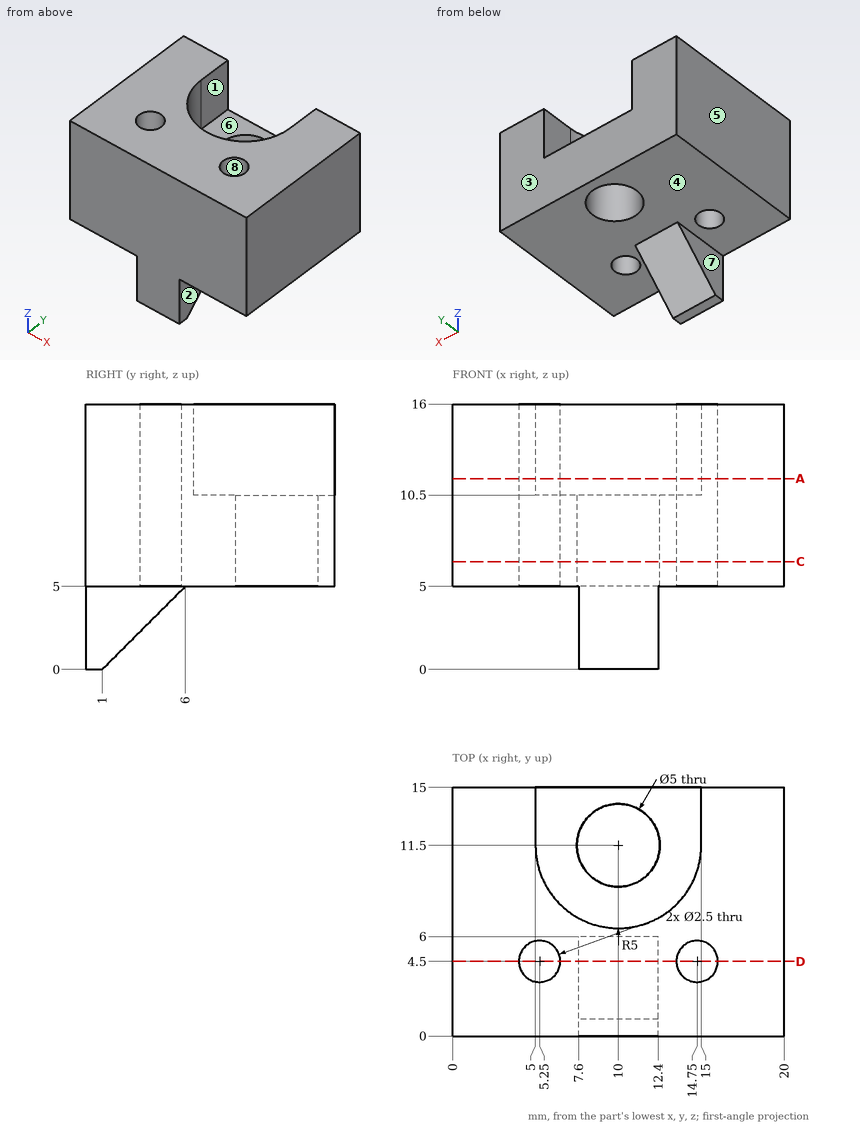
Can you work these out from the drawing? Everything is in mm from the part's minimum corner. A direction names the side the tool comes from. Round coordinates to 2 decimals unless told otherwise and drop trailing zeros. Loops run counter-clockwise (first coordinate to the right, second up) from the corner with the lowest first, then second, coordinate; pieces in that order, holes last. Notation, with made-up numbers: (42, -26) - (60, -26) arc R35 cw to (60, 11) - close; hole circle Ø7 at (-25, 8.25). An arc over 180 degrees is marked (long way). One line per question, with ' | ' between items. Start each with the question number.
Q1. I want a section at A-A (z = 11.5). Write out the boundary of the cut face in (x, y).
Q2. For the marked faces 4, 5, 6, 7 and 8, which set-ups out of +Z, -Z, +X, -X, +Y, -Y let a thin tool reach every point of the face, with its end or its side?
Q3. I want a section at D-D (y = 4.5). Write out the boundary of the cut face in (x, z), then the cut area to 3 significant figures.
Q4. Will these pins go through, and if not, where does the flat tip stop? pin 1 (1.5 mm diameter, centred on x = 5, y = 8, fed in from -Z); pin 2 (2.5 mm diameter, centred on y = 4, z = 2, fed in from +X); pin 3 (4 mm diameter, centred on x = 11.5, y = 9.5, fed in from +Z).
Q5. We'd pull the mould along X, two halves only. Please class the marked faces 1, 2 and 3: +X half, -X half, draft (parallel to the pull), parting line (faces both ways), or undercut.
Q6. I want a section at C-C (z = 6.5). Write out the boundary of the cut face in (x, y), then the cut area to 3 significant figures.
Q7. Please list where these lines run through material, in increasing order: line 1 (X direction, y = 11.5, z = 8.1); line 2 (Y direction, x = 10, z = 6.2); line 3 (Y direction, x = 5.25, z = 9). Write a range as [from, to].
Response values:
1) outline: (0, 0) - (20, 0) - (20, 15) - (15, 15) - (15, 11.5) arc R5 cw to (5, 11.5) - (5, 15) - (0, 15) - close; hole circle Ø2.5 at (5.25, 4.5); hole circle Ø2.5 at (14.75, 4.5)
2) face 4: -Z, +Y | face 5: +Z, -Z, -X, +Y, -Y | face 6: +Z, +Y | face 7: -Z, -X, +Y, -Y | face 8: +Z, -Z
3) outline: (0, 5) - (4, 5) - (4, 16) - (0, 16) - close; (6.5, 5) - (7.6, 5) - (7.6, 3.5) - (12.4, 3.5) - (12.4, 5) - (13.5, 5) - (13.5, 16) - (6.5, 16) - close; (16, 5) - (20, 5) - (20, 16) - (16, 16) - close | area: 172 mm²
4) pin 1: stops at z = 5 | pin 2: stops at x = 12.4 | pin 3: stops at z = 10.5
5) face 1: undercut | face 2: +X half | face 3: draft
6) outline: (0, 0) - (20, 0) - (20, 15) - (0, 15) - close; hole circle Ø2.5 at (5.25, 4.5); hole circle Ø5 at (10, 11.5); hole circle Ø2.5 at (14.75, 4.5) | area: 271 mm²
7) line 1: x = [0, 7.5], [12.5, 20] | line 2: y = [0, 9], [14, 15] | line 3: y = [0, 3.25], [5.75, 15]
